Input: part model. Units: mm. Frame: model coordinates. Face numbers are marked on the shaded views. A direction names the side the tool comes from. Round coordinates to 2 decimals unless told otherwise and drop trailing zeros. Order: outer loops, then holes, each group sorted by start corner. A loop starts at its lowest first (then second) coordinate and runs counter-clockwise, first axis right, second up. Notation, with made-up numbers: M 60.5,61 L 64.5,61 A8 ccw 64.5,75 Z; hole C -23.5,7.25 d11. An arc over 180 degrees is marked long. One line per question, with ' | ' between items.
```python
from build123d import *

# Parameters (mm, degrees)
SKETCH_1_W           = 13
SKETCH_1_H           = 13
SKETCH_1_R           = 2.65
EXTRUDE_1_DEPTH      = 10
EXTRUDE_1_2_DEPTH    = 10
SKETCH_2_R           = 4.5
CUT_EXTRUDE_2_DEPTH  = 5
EXTRUDE_2_DEPTH      = 14.5
EXTRUDE_2_DEPTH_BACK = 14.5
SKETCH_4_W           = 85
SKETCH_4_H           = 10
FILLET_6_R           = 10
SKETCH_9_R           = 3.2
EXTRUDE_3_DEPTH      = 29
CUT_EXTRUDE_6_DEPTH  = 13
CUT_EXTRUDE_7_DEPTH  = 5
SKETCH_12_R          = 1.8
CUT_EXTRUDE_8_DEPTH  = 12


with BuildPart() as part:
    # Sketch 1 → Extrude 1 (new body)
    with BuildSketch(Plane.XY):
        with Locations((-7.792845361, -5.303981357)):
            Rectangle(SKETCH_1_W, SKETCH_1_H)
        with Locations((-7.792845361, -5.303981357)):
            Circle(SKETCH_1_R, mode=Mode.SUBTRACT)
    extrude(amount=EXTRUDE_1_DEPTH)


with BuildPart() as body_2:
    # Sketch 1 → Extrude 1 2 (new body)
    with BuildSketch(Plane.XY):
        Polygon((12.707154639, 1.196018643), (25.707154639, 1.196018643), (25.707154639, -5.303981357), (25.707154639, -11.803981357), (12.707154639, -11.803981357), align=None)
        with Locations((19.207154639, -5.303981357)):
            Circle(SKETCH_1_R, mode=Mode.SUBTRACT)
    extrude(amount=EXTRUDE_1_2_DEPTH)


with BuildPart() as cut_extrude_2_tool:
    # Sketch 2 → Cut-Extrude 2 (new body)
    with BuildSketch(Plane.XY.offset(10)):
        with Locations((-7.792845361, -5.303981357)):
            Circle(SKETCH_2_R)
        with Locations((19.207154639, -5.303981357)):
            Circle(SKETCH_2_R)
    extrude(amount=-CUT_EXTRUDE_2_DEPTH)


with BuildPart() as part_1:
    add(part.part)

    # Cut-Extrude 2: cut by cut_extrude_2_tool
    add(cut_extrude_2_tool.part, mode=Mode.SUBTRACT)



with BuildPart() as body_2_1:
    add(body_2.part)

    # Cut-Extrude 2: cut by cut_extrude_2_tool
    add(cut_extrude_2_tool.part, mode=Mode.SUBTRACT)


with BuildPart() as part_2:
    add(part_1.part)

    add(body_2_1.part)  # Extrude 2 merges body 2
    # Sketch 4 → Extrude 2 (add, two sides: drawn at the far end of the back side and taken through both)
    with BuildSketch(Plane.ZY.offset(-5.707154639).offset(-EXTRUDE_2_DEPTH_BACK)):
        with Locations((42.5, -16.803981357)):
            Rectangle(SKETCH_4_W, SKETCH_4_H)
    extrude(amount=EXTRUDE_2_DEPTH + EXTRUDE_2_DEPTH_BACK)

    # Fillet 6
    # the kernel refuses this fillet: 10 mm, written as the material it adds along each edge
    with BuildSketch(Plane(origin=(20.207154639, -11.803981357, 0), x_dir=(0, -1, 0), z_dir=(0, 0, 1))) as fillet_6_piece_1:
        with BuildLine():
            CenterArc((8.93028555, 10), FILLET_6_R, 206.74368395, 63.25631605)
            Line((0, 5.5), (0, 0))
            Line((0, 0), (8.93028555, 0))
        make_face()
    extrude(amount=10)
    with BuildSketch(Plane(origin=(-8.792845361, -11.803981357, 0), x_dir=(-1, 0, 0), z_dir=(0, 0, 1))) as fillet_6_piece_2:
        with BuildLine():
            CenterArc((10, 8.93028555), FILLET_6_R, 180, 63.25631605)
            Line((0, 8.93028555), (0, 0))
            Line((0, 0), (5.5, 0))
        make_face()
    extrude(amount=10)

    # Sketch 9 → Extrude 3 (add)
    with BuildSketch(Plane.ZY.offset(8.792845361)):
        with BuildLine():
            Line((85, -21.803981357), (100, -21.803981357))
            Line((100, -21.803981357), (100, -4.303981357))
            ThreePointArc((100, -4.303981357), (92.5, 3.196018643), (85, -4.303981357))
            Line((85, -4.303981357), (85, -21.803981357))
        make_face()
        with Locations((92.5, -4.303981357)):
            Circle(SKETCH_9_R, mode=Mode.SUBTRACT)
    extrude(amount=-EXTRUDE_3_DEPTH)

    # Sketch 10 → Cut-Extrude 6 (cut)
    with BuildSketch(Plane.XY.offset(100)):
        Polygon((17.207154639, 3.196018643), (17.207154639, -19.803981357), (17.207154639, -21.803981357), (-5.792845361, -21.803981357), (-5.792845361, -19.803981357), (-5.792845361, 3.196018643), align=None)
    extrude(amount=-CUT_EXTRUDE_6_DEPTH, mode=Mode.SUBTRACT)

    # Sketch 11 → Cut-Extrude 7 (cut)
    with BuildSketch(Plane.XY.offset(87)):
        Polygon((-5.792845361, 3.128632746), (-5.792845361, -9.303981357), (17.207154639, -10.5044716), (17.207154639, 3.128632746), align=None)
    extrude(amount=-CUT_EXTRUDE_7_DEPTH, mode=Mode.SUBTRACT)

    # Sketch 12 → Cut-Extrude 8 (cut)
    with BuildSketch(Plane.XZ.offset(21.803981357)):
        with Locations(Location((5.707154639, 32.798781039, 0), (0, 0, 270))):
            Circle(SKETCH_12_R)
        with Locations((5.707154639, 95.098664418)):
            Circle(SKETCH_12_R)
    extrude(amount=-CUT_EXTRUDE_8_DEPTH, mode=Mode.SUBTRACT)


solid = part_2.part
```
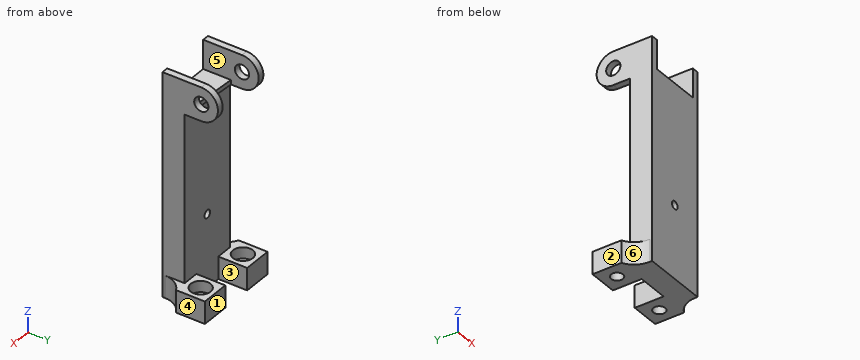
Item 1: Line query: line 1 along Z through (x, y) = (-6.5, -11.5); line 2 along Y through (x, z) = (-7.5, 8); line 3 along Y through (x, z) = (-7.25, 92.5). Output: solid intervals per line, ascending. Write a range as from..to.
Report:
line 1: 0..10, 85..100 | line 2: -21.8..-9.79, -0.81..1.2 | line 3: -21.8..-7.5, -1.1..3.2
Item 2: First-contact query: pin 1 (14 mm diameter, centred on x = 0.5, y = -13, fed in from +Z); pin 2 (8.5 mm diameter, centred on y = -4.3, z = 92.5, fed in from -X); pin 3 (4.5 mm diameter, centred on y = -4, z = 90, fed in from +X); pin 4 (4.5 mm diameter, centred on x = 5.71, z = 32.8, fed in from +Y). Flat tips, straight axial feed; report the tip coordinate or a pass-through.
Report:
pin 1: z = 100 | pin 2: x = -8.79 | pin 3: x = 20.21 | pin 4: y = -11.8
Item 3: Section query C-C, the plane z = 9. Return loops of the section in (x, y).
Report:
outline: M -14.29,-11.8 A10 cw -8.79,-20.73 L -8.79,-21.8 L 20.21,-21.8 L 20.21,-20.73 A10 cw 25.71,-11.8 L 25.71,1.2 L 12.71,1.2 L 12.71,-11.8 L -1.29,-11.8 L -1.29,1.2 L -14.29,1.2 Z; hole C -7.79,-5.3 d9; hole C 19.21,-5.3 d9
Item 4: Section query D-D, the plane z = 39. Return loops of the section in (x, y).
Report:
outline: M -8.79,-21.8 L 20.21,-21.8 L 20.21,-11.8 L -8.79,-11.8 Z
Item 5: Section query A-A, the plane z = 92.5. Return loops of the section in (x, y).
Report:
outline: M -8.79,-21.8 L -5.79,-21.8 L -5.79,-7.5 L -8.79,-7.5 Z; M -8.79,-1.1 L -5.79,-1.1 L -5.79,3.2 L -8.79,3.2 Z; M 17.21,-21.8 L 20.21,-21.8 L 20.21,-7.5 L 17.21,-7.5 Z; M 17.21,-1.1 L 20.21,-1.1 L 20.21,3.2 L 17.21,3.2 Z
Item 6: Section query B-B, the plane y = -13. Return loops of the section in (x, z), plus the area to 3 significant figures.
Report:
outline: M -12.45,0 L 23.87,0 L 23.87,10 L 20.21,10 L 20.21,100 L 17.21,100 L 17.21,87 L -5.79,87 L -5.79,100 L -8.79,100 L -8.79,10 L -12.45,10 Z; hole C 5.71,32.8 d3.6 | area: 2,660 mm²
Item 7: Access query for the marked faces 1, 2 and 3. Directions: +Z, -Z, +X, -X, +Y, -Y. A direction counts if a zero-diameter tool reaches every point of the face in a straight line with its end or side. Return the directions, or none.
Report:
face 1: -Z, +X, -X, +Y | face 2: +Z, -Z, -X, +Y, -Y | face 3: -Z, +Y
Item 8: Mould query, pull axis X, two halves, no side actions, for the marked faces 4, 5 and 6. Classes: +X half, -X half, draft (parallel to the pull), parting line (faces both ways), or undercut.
Report:
face 4: +X half | face 5: undercut | face 6: -X half
